CAD build for the part. Positions are in the model's coordinates, mm. A direction names the side the tool comes from. Give positions to 0.01 mm unless a question says otherwise; leave off trailing zeros. Loops run counter-clockwise (first coordinate to the right, second up) from the corner with the lowest first, then second, coordinate; pieces in that order, holes last. Notation, with made-up numbers: (16.5, 42) - (72.5, 42) arc R23 cw to (72.5, 67) - close; hole circle Ø10 at (37.25, 84.5). An arc over 180 degrees is marked (long way). Return JSON: item names as keys, results as strings.
from build123d import *

# Parameters (mm, degrees)
BASE_FLANGE1_DEPTH = 296
SKETCH2_W          = 2.75
SKETCH2_H          = 20.5
CUT_EXTRUDE1_DEPTH = 13


# Sheet-metal steps are written as plain solids
with BuildPart() as part:
    # Sketch1 → Base-Flange1 (new body)
    with BuildSketch(Plane.XY):
        with BuildLine():
            Line((0, 0), (0, 18.0634))
            ThreePointArc((0, 18.0634), (-0.567217008, 19.432782992), (-1.9366, 20))
            Line((-1.9366, 20), (-40, 20))
            Line((-40, 20), (-40, 18.8))
            Line((-40, 18.8), (-1.9366, 18.8))
            ThreePointArc((-1.9366, 18.8), (-1.415745145, 18.584254855), (-1.2, 18.0634))
            Line((-1.2, 18.0634), (-1.2, 0))
            Line((-1.2, 0), (0, 0))
        make_face()
    extrude(amount=BASE_FLANGE1_DEPTH)

    # Sketch2 → Cut-Extrude1 (cut)
    with BuildSketch(Plane(origin=(0, 0, 0), x_dir=(0, 0, -1), z_dir=(1, 0, 0))):
        with Locations((-119.558385949, 9.989549108)):
            Rectangle(SKETCH2_W, SKETCH2_H)
    extrude(amount=-CUT_EXTRUDE1_DEPTH, mode=Mode.SUBTRACT)


solid = part.part
1. Cut at D-D, the plane x = -34. Write the cut outline in (y, z).
Values follow:
{"outline": "(18.8, 0) - (20, 0) - (20, 296) - (18.8, 296) - close"}
2. Drill centre lines: probe 1 along Y at (x, z) = (-8, 181); probe 2 along X at (y, z) = (5.5, 192.5). Where is each one in solid material? Low to high.
Values follow:
{"probe 1": "y = 18.8 to 20", "probe 2": "x = -1.2 to 0"}
3. Cut at C-C, the plane z = 160. Write the cut outline in (x, y).
Values follow:
{"outline": "(-40, 18.8) - (-1.94, 18.8) arc R0.74 cw to (-1.2, 18.06) - (-1.2, 0) - (0, 0) - (0, 18.06) arc R1.94 ccw to (-1.94, 20) - (-40, 20) - close"}
4. Drop flat-ended pins along their axis: P1, Ø1, axis at x = -15.5, z = 160.5, coming from the -Y side; P2, Ø10.5, axis at x = -7, y = 10, coming from the -Z side; P3, Ø10, axis at y = 11.5, z = 241, coming from the -X side; P4, Ø1.3, axis at y = 19, z = 119, coming from the +X side. Give the stop position or say it passes through.
Values follow:
{"P1": "stops at y = 18.8", "P2": "passes through", "P3": "stops at x = -1.2", "P4": "stops at x = -13"}
5. Which spindle directions (+Z, -Z, +X, -X, +Y, -Y) get a long thin tool onto all of the face, cutting with end or side? Do faces 1 (the face through (-1.2, 9, 58)), 2 (the face through (-14, 19, 296)), 3 (the face through (-1, 12, 120.933)). Say none if no direction does.
Values follow:
{"face 1": "+Z, -Z, -X, -Y", "face 2": "+Z, +X, -X, +Y, -Y", "face 3": "+X, +Y, -Y"}
6. Cut at A-A, the plane y = 7.25. Write the cut outline in (x, z).
Values follow:
{"outline": "(-1.2, 0) - (0, 0) - (0, 118.18) - (-1.2, 118.18) - close; (-1.2, 120.93) - (0, 120.93) - (0, 296) - (-1.2, 296) - close"}
7. Cut at B-B, the plane x = -8. Write the cut outline in (y, z), plus the area to 3 significant figures.
Values follow:
{"outline": "(18.8, 0) - (20, 0) - (20, 118.18) - (18.8, 118.18) - close; (18.8, 120.93) - (20, 120.93) - (20, 296) - (18.8, 296) - close", "area": "352 mm²"}
